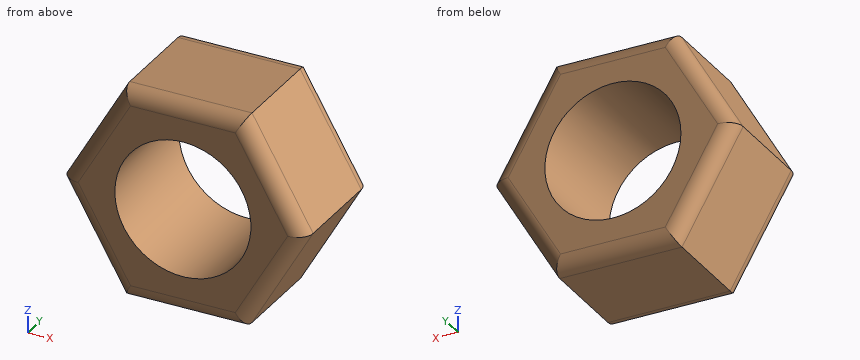
Autodesk Inventor part; units mm, degrees
ref_plane "YZ Plane" through (0, 0, 0) normal (1, 0, 0) x (0, 1, 0)
ref_plane "XZ Plane" through (0, 0, 0) normal (0, 1, 0) x (-1, 0, 0)
ref_plane "XY Plane" through (0, 0, 0) normal (0, 0, 1) x (1, 0, 0)
sketch "Sketch1" plane through (0, 0, 0) normal (0, 1, 0) x (-1, 0, 0)
  line L0 (-0.4861, -7.0529) -> (-8.569, -7.0529)
  line L1 (-8.569, -7.0529) -> (-12.6104, -0.0529)
  line L2 (-12.6104, -0.0529) -> (-8.569, 6.9471)
  line L3 (-8.569, 6.9471) -> (-0.4861, 6.9471)
  line L4 (-0.4861, 6.9471) -> (3.5554, -0.0529)
  line L5 (3.5554, -0.0529) -> (-0.4861, -7.0529)
  circle A0 centre (-4.5275, -0.0529) radius 4.5
  dimension "d0" = 14
  dimension "d1" = 9
extrude "Extrusion1" add sketch "Sketch1" along normal blind 8
fillet "Fillet1" radius 1 12 edges at (4.5275, 8, 6.9471) (10.5897, 8, 3.4471) (10.5897, 8, -3.5529) (4.5275, 8, -7.0529) (-1.5346, 8, -3.5529) (-1.5346, 8, 3.4471) (4.5275, 0, 6.9471) (10.5897, 0, 3.4471) (10.5897, 0, -3.5529) (4.5275, 0, -7.0529) (-1.5346, 0, -3.5529) (-1.5346, 0, 3.4471)
properties part number "Tuerca"
Design review of the part built by this model. Coordinates are the model's own, in mm. Give positions to 0.01 mm unless a question says otherwise; leave off trailing zeros. Loops run counter-clockwise (first coordinate to the right, second up) from the corner with the lowest first, then second, coordinate; pieces in that order, holes last. Notation, with made-up numbers: (68, 21.25) -> (72, 21.25) arc R15 cw to (72, 31.25) -> close; hole circle Ø9 at (-25.75, 53.5). An arc over 180 degrees is marked (long way). One line per item, written item: value.
Q1. We need section B-B on x = 4.5. Give the boundary of the cut face in (y, z), and give its area (3 significant figures).
Numbers:
outline: (0, -6.05) arc R1 ccw to (1, -7.05) -> (7, -7.05) arc R1 ccw to (8, -6.05) -> (8, -4.55) -> (0, -4.55) -> close; (0, 4.45) -> (8, 4.45) -> (8, 5.95) arc R1 ccw to (7, 6.95) -> (1, 6.95) arc R1 ccw to (0, 5.95) -> close
area: 39.1 mm^2
Q2. For L1, parallel to X at y = 2.75, z = -3.25; L2, parallel to Z at x = 7.25, y = 3.75; L3, parallel to X at y = 5.25, z = 1, list the stretches that pass through material, from the lowest coordinate up.
Numbers:
L1: x = -1.71 to 1.36, 7.69 to 10.76
L2: z = -7.05 to -3.64, 3.53 to 6.95
L3: x = -2.95 to 0.15, 8.9 to 12
Q3. For pin 1 Ø4 at (y, z) = (3.5, 0.5) entering from +X, flat-tipped, find the tip position at first contact; note if it passes through.
Numbers:
pin 1: stops at x = 12.61
Q4. We need section A-A on y = 4.5. Give the boundary of the cut face in (x, z).
Numbers:
outline: (-3.56, -0.05) -> (0.49, -7.05) -> (8.57, -7.05) -> (12.61, -0.05) -> (8.57, 6.95) -> (0.49, 6.95) -> close; hole circle Ø9 at (4.53, -0.05)
